The listing builds one solid part. Answer for the finished solid, in the listing's coordinates (mm). Face numbers are marked on the shaded views. A direction names the side the tool comes from. Round coordinates to 2 decimals unless told otherwise and drop trailing zeros. Loops run counter-clockwise (first coordinate to the right, second up) from the corner with the lowest first, then second, coordinate; pieces in that order, holes last. Notation, with made-up numbers: (84.25, 89.5) - (106.25, 89.5) arc R33 cw to (106.25, 124.5) - close; hole circle Ø1 at (25.25, 5.5). An arc over 180 degrees is marked (long way). One line per question, with ' | ' between items. Start each with the question number.
from build123d import *

# Parameters (mm, degrees)
F1_DEPTH        = 11
F5_COPIES_COUNT = 3
F6_SIZE         = 2
F7_SIZE         = 2


# Not quite as in the source:
# - a pattern or mirror of a feature is missing from the dataset's text; its kind, count and spacing are read off the source's solid


with BuildPart() as f1:
    # F0 (on Top) → F1 (new body)
    with BuildSketch(Plane.XY):
        with BuildLine():
            ThreePointArc((2.4931063701, -26.2757839441), (9.6114548877, -16.6475282001), (21.5089432149, -15.2969854229))
            ThreePointArc((21.5089432149, -15.2969854229), (42.1995974306, 0), (21.5089432149, 15.2969854229))
            ThreePointArc((21.5089432149, 15.2969854229), (9.6114548877, 16.6475282001), (2.4931063701, 26.2757839441))
            ThreePointArc((2.4931063701, 26.2757839441), (-21.0997987153, 36.5459234044), (-24.002049585, 10.9787985212))
            ThreePointArc((-24.002049585, 10.9787985212), (-19.2229097754, 0), (-24.002049585, -10.9787985212))
            ThreePointArc((-24.002049585, -10.9787985212), (-21.0997987153, -36.5459234044), (2.4931063701, -26.2757839441))
        make_face()
    extrude(amount=F1_DEPTH)

    # F2 (on Right) → F3 (revolve, cut)
    with BuildSketch(Plane.YZ):
        Polygon((0, 11), (0, 0), (10, 0), (10, 1.8), (11, 1.8), (11, 9.1), (10.5, 9.1), (11, 11), align=None)
    revolve(axis=Axis((0, 0, 3.7751235068), (0, 0, -1)), mode=Mode.SUBTRACT)

    # F4 (on Front) → F5 (revolve, cut)
    with BuildSketch(Plane.XZ):
        Polygon((16, 0), (27, 0), (27, 11), (16, 11), (16, 8.3), (14.3, 8.3), (14.3, 2.2), (16, 2.2), align=None)
    f5 = revolve(axis=Axis((27, 0, 6.29213918), (0, 0, -1)), mode=Mode.SUBTRACT)

    # F5_copies: F5 ×3 about axis
    f5_copies_axis = Axis((0, 0, 0), (0, 0, 1))
    for i in range(1, F5_COPIES_COUNT):
        add(f5.rotate(f5_copies_axis, i * 360 / F5_COPIES_COUNT), mode=Mode.SUBTRACT)

    # F6
    f6_edges = [f1.edges().sort_by_distance(p)[0] for p in [
        (9.611455, -16.647528, 11),
    ]]
    chamfer(f6_edges, length=F6_SIZE)

    # F7
    f7_edges = [f1.edges().sort_by_distance(p)[0] for p in [
        (9.611455, -16.647528, 0),
        (-21.099799, -36.545923, 0),
        (-19.22291, 0, 0),
        (-21.099799, 36.545923, 0),
        (42.199597, 0, 0),
        (9.611455, 16.647528, 0),
    ]]
    chamfer(f7_edges, length=F7_SIZE)


solid = f1.part
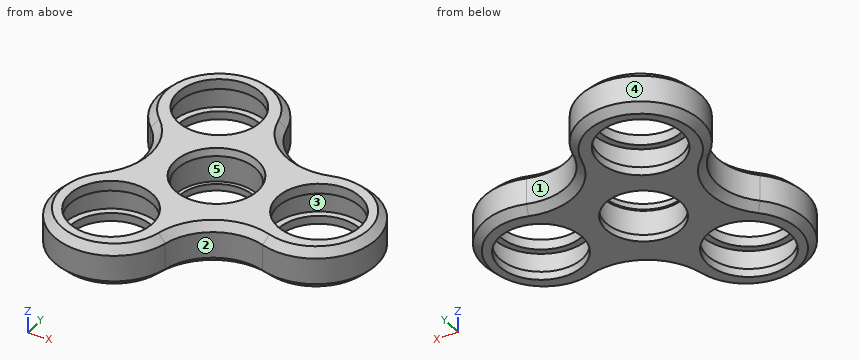
(1) Find section B-B on z = 5. Write down the section's boundary in (x, y), plus the area to 3 significant figures.
(2) Find section A-A on y = 0. Count the separate pieces of the cut face and the enclosed holes in it, plus the area to 3 significant figures.
(3) A tool of negligible diameter and unlimited length cuts with its end or side. For the marked faces 4 and 5, from which of +Z, -Z, +X, -X, +Y, -Y can it reach the whole face along a straight path? Write none if from no direction.
(4) Each of these flat-tipped pins is pushed along its axis until it touches: P1, Ø15, axis at x = -13.5, y = 23.38, coming from the +Z side; P2, Ø1, axis at x = 12, z = 6.5, coming from the -Y side; P3, Ø1.5, axis at y = 19.5, z = 8, coming from the +X side; P4, Ø1.5, axis at y = -29, z = 7.5, coming from the +X side. Where does it stop, or does it pass through?
(5) Consider L1, parallel to X at y = -8, z = 10.75; L2, parallel to Y at x = 26, z = 2.5; L3, parallel to Y at x = -15, z = 10.25. Determine where each line is inside the solid, lowest interval first.
(6) Determine the mould class of the marked faces 1, 2 and 3 for opening direction Y: pulls with the +Y half, pulls with the -Y half, needs draft (parallel to the pull), parting line crosses it, or undercut.
Answer below:
1) outline: (-24, -10.98) arc R16 ccw (long way) to (2.49, -26.28) arc R15 cw to (21.51, -15.3) arc R16 ccw (long way) to (21.51, 15.3) arc R15 cw to (2.49, 26.28) arc R16 ccw (long way) to (-24, 10.98) arc R15 cw to start; hole circle Ø25.4 at (-13.5, -23.38); hole circle Ø25.4 at (-13.5, 23.38); hole circle Ø22 at (0, 0); hole circle Ø25.4 at (27, 0) | area: 1,310 mm2
2) separate pieces: 3 | enclosed holes: 0 | area: 167 mm2
3) face 4: +Z, -Z | face 5: none
4) P1: through | P2: y = -15.73 | P3: x = 6.79 | P4: x = 1.9
5) L1: -19.51 to -7.45, 7.45 to 19.45, 34.55 to 37.99 | L2: -16 to -12.66, 12.66 to 16 | L3: -37.32 to -34.28, -12.49 to 12.49, 34.28 to 37.32
6) face 1: pulls with the +Y half | face 2: pulls with the -Y half | face 3: undercut
